Build history of the part. All positions in model axes, mm. Face numbers are marked on the shaded views. A direction names the side the tool comes from. Give positions to 0.01 mm unless a question says otherwise; leave off trailing zeros. Order: outer loops, then holes, each group sorted by start corner. A loop starts at its lowest first (then second) coordinate and runs counter-clockwise, first axis right, second up. Notation, with made-up numbers: M -32.5,66 L 1.5,66 A14 cw 1.5,73 Z; hole C -7,14 d8. An arc over 180 degrees is marked long. Answer as CSV lines item,"result".
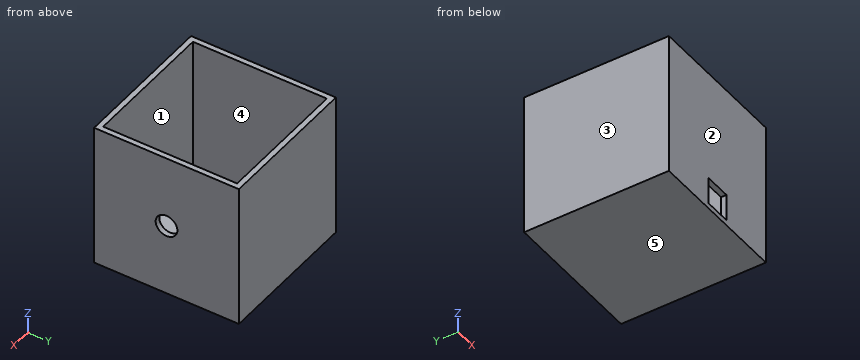
from build123d import *

# Parameters (mm, degrees)
F0_W     = 80
F0_H     = 80
F1_DEPTH = 3
F3_DEPTH = 74
F4_W     = 80
F4_H     = 80
F5_DEPTH = 3
F6_R     = 6
F7_DEPTH = 3
F8_W     = 15
F8_H     = 15
F9_DEPTH = 3


with BuildPart() as f1:
    # F0 (on Front) → F1 (new body)
    with BuildSketch(Plane.XZ):
        Rectangle(F0_W, F0_H)
    extrude(amount=F1_DEPTH)

    # F2 (on face) → F3 (join)
    with BuildSketch(Plane(origin=(0, 0, 0), x_dir=(-1, 0, 0), z_dir=(0, 1, 0))):
        Polygon((-40, -40), (40, -40), (40, 40), (37, 40), (37, 37), (37, -37), (-37, -37), (-37, 37), (-37, 40), (-40, 40), align=None)
    extrude(amount=F3_DEPTH)

    # F4 (on face) → F5 (join)
    with BuildSketch(Plane(origin=(0, 74, 0), x_dir=(-1, 0, 0), z_dir=(0, 1, 0))):
        Rectangle(F4_W, F4_H)
    extrude(amount=F5_DEPTH)

    # F6 (on face) → F7 (cut)
    with BuildSketch(Plane.YZ.offset(40)):
        with Locations((37, 0)):
            Circle(F6_R)
    extrude(amount=-F7_DEPTH, mode=Mode.SUBTRACT)

    # F8 (on face) → F9 (cut)
    with BuildSketch(Plane.XZ.offset(3)):
        with Locations((0, -29.5)):
            Rectangle(F8_W, F8_H)
    extrude(amount=-F9_DEPTH, mode=Mode.SUBTRACT)


solid = f1.part
Item 1: Pull direction Y, two halves, no side cores. Call the marked faces 1, 2 and 3: released by +Y, released by -Y, zero draft, split by the parting line, or undercut.
Geometry says:
face 1,"undercut"
face 2,"released by -Y"
face 3,"zero draft"
Item 2: Band-saw the part on C-C (z = 12.5). Give the cut face in (x, y).
Geometry says:
outline,"M -40,-3 L 40,-3 L 40,77 L -40,77 Z; hole M -37,0 L 37,0 L 37,74 L -37,74 Z"
Item 3: Band-saw the part on A-A (y = 37). Give the cut face in (x, z), and give its area (3 significant figures).
Geometry says:
outline,"M -40,-40 L 40,-40 L 40,-6 L 37,-6 L 37,-37 L -37,-37 L -37,40 L -40,40 Z; M 37,6 L 40,6 L 40,40 L 37,40 Z"
area,"666 mm2"
Item 4: Drop a flat-ended pin along its axis: pin 1 (1.5 mm diameter, centred on x = 13, y = 58, fed in from +Z). Give the stop position or say it passes through.
Geometry says:
pin 1,"stops at z = -37"
Item 5: Band-saw the part on B-B (x = -3.5). Give the cut face in (y, z), and give its area (3 significant figures).
Geometry says:
outline,"M -3,-40 L 77,-40 L 77,40 L 74,40 L 74,-37 L -3,-37 Z; M -3,-22 L 0,-22 L 0,40 L -3,40 Z"
area,"657 mm2"
Item 6: Probe line 1 along X through (y, z) = (38.5, 22); line 2 along Y through (x, z) = (27, 23); line 3 along Z through (x, y) = (38.3, 37). List the from-to ranges inside material, lowest first. Write a range as from..to.
Geometry says:
line 1,"x = -40..-37, 37..40"
line 2,"y = -3..0, 74..77"
line 3,"z = -40..-6, 6..40"
Item 7: 3-axis set-ups, long thin cutter, end or side, ignore diameter. For the marked faces 4 and 5: which of +Z, -Z, +X, -X, +Y, -Y reach the whole face in a straight line?
Geometry says:
face 4,"+Z"
face 5,"-Z, +X, -X, +Y, -Y"
Item 8: Band-saw the part on D-D (y = 50.5). Give the cut face in (x, z).
Geometry says:
outline,"M -40,-40 L 40,-40 L 40,40 L 37,40 L 37,-37 L -37,-37 L -37,40 L -40,40 Z"
